```python
from build123d import *

# Parameters (mm, degrees)
F0_W     = 15
F0_H     = 15
F0_R     = 0.5
F1_DEPTH = 1
F2_DEPTH = 5


with BuildPart() as f1:
    # F0 (on Top) → F1 (new body)
    with BuildSketch(Plane.XY):
        Rectangle(F0_W, F0_H)
        with Locations((-6, -6)):
            Circle(F0_R, mode=Mode.SUBTRACT)
        with Locations((-4, -6)):
            Circle(F0_R, mode=Mode.SUBTRACT)
        with Locations((-6, -4)):
            Circle(F0_R, mode=Mode.SUBTRACT)
        with Locations((-4, -4)):
            Circle(F0_R, mode=Mode.SUBTRACT)
        with Locations((-2, -6)):
            Circle(F0_R, mode=Mode.SUBTRACT)
        with Locations((-2, -4)):
            Circle(F0_R, mode=Mode.SUBTRACT)
        with Locations((-6, -2)):
            Circle(F0_R, mode=Mode.SUBTRACT)
        with Locations((-4, -2)):
            Circle(F0_R, mode=Mode.SUBTRACT)
        with Locations((-2, -2)):
            Circle(F0_R, mode=Mode.SUBTRACT)
        with Locations((0, -6)):
            Circle(F0_R, mode=Mode.SUBTRACT)
        with Locations((2, -6)):
            Circle(F0_R, mode=Mode.SUBTRACT)
        with Locations((0, -4)):
            Circle(F0_R, mode=Mode.SUBTRACT)
        with Locations((2, -4)):
            Circle(F0_R, mode=Mode.SUBTRACT)
        with Locations((4, -6)):
            Circle(F0_R, mode=Mode.SUBTRACT)
        with Locations((6, -6)):
            Circle(F0_R, mode=Mode.SUBTRACT)
        with Locations((4, -4)):
            Circle(F0_R, mode=Mode.SUBTRACT)
        with Locations((6, -4)):
            Circle(F0_R, mode=Mode.SUBTRACT)
        with Locations((0, -2)):
            Circle(F0_R, mode=Mode.SUBTRACT)
        with Locations((2, -2)):
            Circle(F0_R, mode=Mode.SUBTRACT)
        with Locations((4, -2)):
            Circle(F0_R, mode=Mode.SUBTRACT)
        with Locations((6, -2)):
            Circle(F0_R, mode=Mode.SUBTRACT)
        with Locations((-6, 0)):
            Circle(F0_R, mode=Mode.SUBTRACT)
        with Locations((-4, 0)):
            Circle(F0_R, mode=Mode.SUBTRACT)
        with Locations((-6, 2)):
            Circle(F0_R, mode=Mode.SUBTRACT)
        with Locations((-4, 2)):
            Circle(F0_R, mode=Mode.SUBTRACT)
        with Locations((-2, 0)):
            Circle(F0_R, mode=Mode.SUBTRACT)
        with Locations((-2, 2)):
            Circle(F0_R, mode=Mode.SUBTRACT)
        with Locations((-6, 4)):
            Circle(F0_R, mode=Mode.SUBTRACT)
        with Locations((-4, 4)):
            Circle(F0_R, mode=Mode.SUBTRACT)
        with Locations((-6, 6)):
            Circle(F0_R, mode=Mode.SUBTRACT)
        with Locations((-4, 6)):
            Circle(F0_R, mode=Mode.SUBTRACT)
        with Locations((-2, 4)):
            Circle(F0_R, mode=Mode.SUBTRACT)
        with Locations((-2, 6)):
            Circle(F0_R, mode=Mode.SUBTRACT)
        Circle(F0_R, mode=Mode.SUBTRACT)
        with Locations((2, 0)):
            Circle(F0_R, mode=Mode.SUBTRACT)
        with Locations((0, 2)):
            Circle(F0_R, mode=Mode.SUBTRACT)
        with Locations((2, 2)):
            Circle(F0_R, mode=Mode.SUBTRACT)
        with Locations((4, 0)):
            Circle(F0_R, mode=Mode.SUBTRACT)
        with Locations((6, 0)):
            Circle(F0_R, mode=Mode.SUBTRACT)
        with Locations((4, 2)):
            Circle(F0_R, mode=Mode.SUBTRACT)
        with Locations((6, 2)):
            Circle(F0_R, mode=Mode.SUBTRACT)
        with Locations((0, 4)):
            Circle(F0_R, mode=Mode.SUBTRACT)
        with Locations((2, 4)):
            Circle(F0_R, mode=Mode.SUBTRACT)
        with Locations((0, 6)):
            Circle(F0_R, mode=Mode.SUBTRACT)
        with Locations((2, 6)):
            Circle(F0_R, mode=Mode.SUBTRACT)
        with Locations((4, 4)):
            Circle(F0_R, mode=Mode.SUBTRACT)
        with Locations((6, 4)):
            Circle(F0_R, mode=Mode.SUBTRACT)
        with Locations((4, 6)):
            Circle(F0_R, mode=Mode.SUBTRACT)
        with Locations((6, 6)):
            Circle(F0_R, mode=Mode.SUBTRACT)
    extrude(amount=F1_DEPTH)

    # F0 (on Top) → F2 (join)
    with BuildSketch(Plane.XY):
        with Locations((-6, 6)):
            Circle(F0_R)
        with Locations((-4, 6)):
            Circle(F0_R)
        with Locations((-2, 6)):
            Circle(F0_R)
        with Locations((0, 6)):
            Circle(F0_R)
        with Locations((2, 6)):
            Circle(F0_R)
        with Locations((4, 6)):
            Circle(F0_R)
        with Locations((6, 6)):
            Circle(F0_R)
        with Locations((6, 4)):
            Circle(F0_R)
        with Locations((4, 4)):
            Circle(F0_R)
        with Locations((2, 4)):
            Circle(F0_R)
        with Locations((0, 4)):
            Circle(F0_R)
        with Locations((-2, 4)):
            Circle(F0_R)
        with Locations((-4, 4)):
            Circle(F0_R)
        with Locations((-6, 4)):
            Circle(F0_R)
        with Locations((-6, 2)):
            Circle(F0_R)
        with Locations((-4, 2)):
            Circle(F0_R)
        with Locations((-2, 2)):
            Circle(F0_R)
        with Locations((0, 2)):
            Circle(F0_R)
        with Locations((2, 2)):
            Circle(F0_R)
        with Locations((4, 2)):
            Circle(F0_R)
        with Locations((6, 2)):
            Circle(F0_R)
        with Locations((6, 0)):
            Circle(F0_R)
        with Locations((4, 0)):
            Circle(F0_R)
        with Locations((2, 0)):
            Circle(F0_R)
        Circle(F0_R)
        with Locations((-2, 0)):
            Circle(F0_R)
        with Locations((-4, 0)):
            Circle(F0_R)
        with Locations((-6, 0)):
            Circle(F0_R)
        with Locations((-6, -2)):
            Circle(F0_R)
        with Locations((-4, -2)):
            Circle(F0_R)
        with Locations((-2, -2)):
            Circle(F0_R)
        with Locations((0, -2)):
            Circle(F0_R)
        with Locations((2, -2)):
            Circle(F0_R)
        with Locations((4, -2)):
            Circle(F0_R)
        with Locations((6, -2)):
            Circle(F0_R)
        with Locations((6, -4)):
            Circle(F0_R)
        with Locations((4, -4)):
            Circle(F0_R)
        with Locations((2, -4)):
            Circle(F0_R)
        with Locations((0, -4)):
            Circle(F0_R)
        with Locations((-2, -4)):
            Circle(F0_R)
        with Locations((-4, -4)):
            Circle(F0_R)
        with Locations((-6, -4)):
            Circle(F0_R)
        with Locations((-6, -6)):
            Circle(F0_R)
        with Locations((-4, -6)):
            Circle(F0_R)
        with Locations((-2, -6)):
            Circle(F0_R)
        with Locations((0, -6)):
            Circle(F0_R)
        with Locations((2, -6)):
            Circle(F0_R)
        with Locations((4, -6)):
            Circle(F0_R)
        with Locations((6, -6)):
            Circle(F0_R)
    extrude(amount=F2_DEPTH)


solid = f1.part
```
Input: part model. Units: mm. Frame: model coordinates. A direction names the side the tool comes from. Coordinates: 2 decimals unless noted, no trailing zeros. Loops run counter-clockwise (first coordinate to the right, second up) from the corner with the lowest first, then second, coordinate; pieces in that order, holes last. Notation, with made-up numbers: M 82,-9 L 108,-9 A17 cw 108,12 Z; hole C 20,-39.5 d4. An arc over 180 degrees is marked long. One line per item, written item: value.
(1) Section C-C (z = 4.1). Give the number of separate pieces and of enclosed holes in the cut face, and give its area (3 significant figures).
Filled in:
separate pieces: 49
enclosed holes: 0
area: 38.5 mm^2
(2) Pin query (flat end, axial travel): pin 1 (1.5 mm diameter, centred on y = 5.5, z = 3.5, fed in from -X); pin 2 (3 mm diameter, centred on x = -5, z = 4, fed in from -Y); pin 3 (2 mm diameter, centred on x = -5.5, z = 3.5, fed in from +Y). Return the tip coordinate at first contact, or that it passes through.
Filled in:
pin 1: x = -6.5
pin 2: y = -6.5
pin 3: y = 6.5
(3) Pull-direction query (X, two-part tool) for faces 3 (the cylindrical face through (1.6, 2.3, 3)), 4 (the flat face through (-4, -4, 5)); classes: +X half, -X half, draft (parallel to the pull), parting line (faces both ways), or undercut.
Filled in:
face 3: undercut
face 4: draft
(4) Reachability of faces 1 (the cylindrical face through (5.5, -2, 3)), 2 (the flat face through (6, 0, 5)) from +Z, -Z, +X, -X, +Y, -Y: full face, straight path, thin tool, end or side. Return the list, or none.
Filled in:
face 1: +Z
face 2: +Z, +X, -X, +Y, -Y
(5) Line query: line 1 along Z through (x, y) = (-1, -3). Output: solid intervals per line, ascending. Write a range as from..to.
Filled in:
line 1: 0..1
(6) Section D-D (y = -4.75). Output: boundary loops of the cut face in (x, z), and give its area (3 significant figures).
Filled in:
outline: M -7.5,0 L 7.5,0 L 7.5,1 L -7.5,1 Z
area: 15.0 mm^2
